Answer from the drawing. Dimensions are ordinates in mm from the lowest x, y and z of the part. A direction names the side the tool comes from. Coordinates: 2 decimals unless noted, no trailing zeros. Loops run counter-clockwise (first coordinate to the right, second up) from the corner with the lowest first, then second, coordinate; pieces in that order, holes last. Notation, with made-up numbers: M 10,39.25 L 69,39.25 A16 ccw 69,63.25 Z; hole C 19,41 d5. An arc over 180 degrees is marked long. Put each result on its own line as item: value.
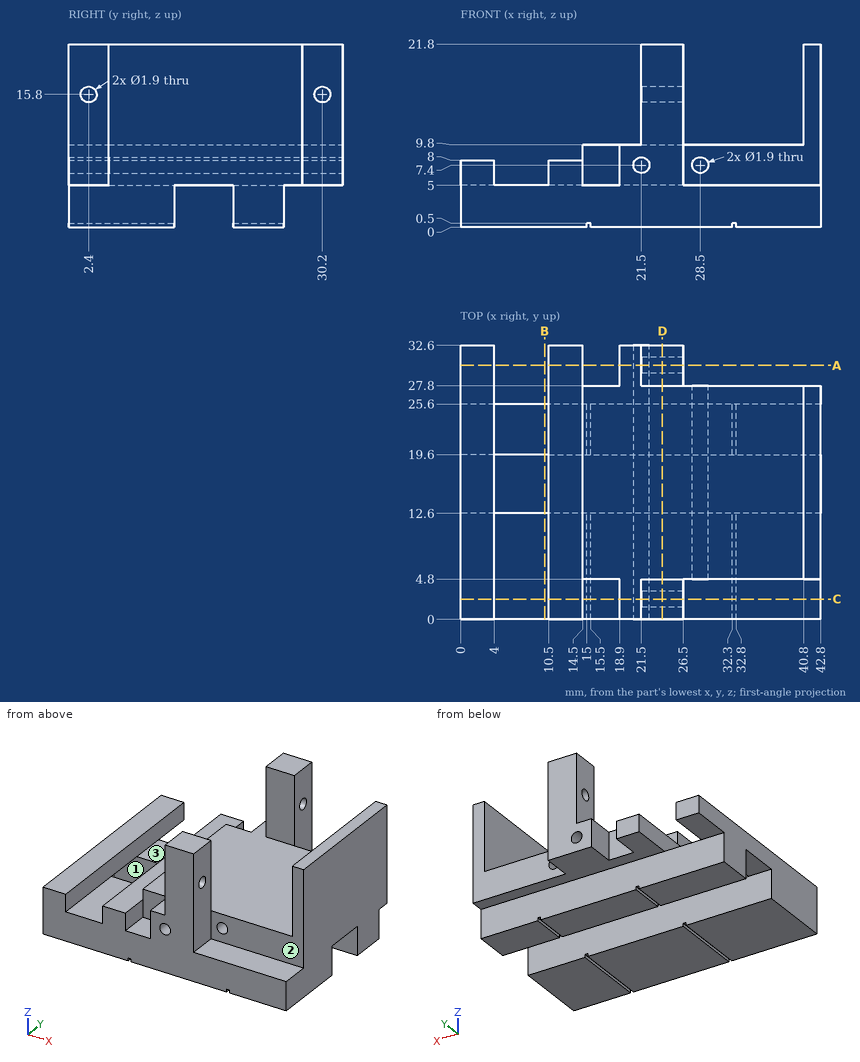
1) Find section C-C, the plane y = 2.4. Count the separate pieces of the cut face and the enclosed holes in it, plus the area to 3 significant figures.
Answer list:
separate pieces: 2
enclosed holes: 1
area: 322 mm^2
2) Find section D-D, the plane x = 24. Write down the section's boundary in (y, z), plus the area to 3 significant figures.
Answer list:
outline: M 0,0 L 12.6,0 L 12.6,5 L 19.6,5 L 19.6,0 L 25.6,0 L 25.6,5 L 32.6,5 L 32.6,21.8 L 27.8,21.8 L 27.8,9.8 L 4.8,9.8 L 4.8,21.8 L 0,21.8 Z; hole C 2.4,15.8 d1.9; hole C 30.2,15.8 d1.9
area: 359 mm^2
3) Find section A-A, the plane y = 30.2. Write down the section's boundary in (x, z).
Answer list:
outline: M 0,5 L 4,5 L 4,8 L 0,8 Z; M 10.5,5 L 14.5,5 L 14.5,8 L 10.5,8 Z; M 18.9,5 L 26.5,5 L 26.5,14.85 L 21.5,14.85 L 21.5,9.8 L 18.9,9.8 Z; M 21.5,16.75 L 26.5,16.75 L 26.5,21.8 L 21.5,21.8 Z; hole C 21.5,7.4 d1.9
4) Given pin 1 Ø6.5 at (x, y) = (6.5, 22.5) entering from +Z; pin 2 Ø4 at (y, z) = (30, 18.5) entering from -X; pin 3 Ø1.5 at (x, z) = (21.5, 7.4) entering from +Y; pin 4 Ø1.5 at (x, y) = (15.5, 21.5) entering from +Z, each flat-ended and moving along its own axis, determine where each tip first touches the part or whether it passes through.
Answer list:
pin 1: stops at z = 8
pin 2: stops at x = 21.5
pin 3: passes through
pin 4: stops at z = 9.8
5) Which of the six approach directions +Z, -Z, +X, -X, +Y, -Y give full straight-line access (tool end or side, diameter ignored) to the marked faces 1, 2 and 3?
Answer list:
face 1: -Z, +X, -X
face 2: +Z, +X, -Y
face 3: +Z, +Y, -Y
6) Find section B-B, the plane x = 10. Write down the section's boundary in (y, z).
Answer list:
outline: M 0,0 L 12.6,0 L 12.6,5 L 0,5 Z; M 19.6,0 L 25.6,0 L 25.6,5 L 19.6,5 Z
7) Straight lines are drawn through the part: line 1 (Y direction, x = 25.1, z = 15.8); line 2 (Z direction, x = 21.5, y = 13); line 3 (Y direction, x = 10.5, z = 1.25). For each, find the intervals that lie inside material, in ascending order. Write a range as [from, to].
Answer list:
line 1: y = [0, 1.45], [3.35, 4.8], [27.8, 29.25], [31.15, 32.6]
line 2: z = [5, 6.45], [8.35, 9.8]
line 3: y = [0, 12.6], [19.6, 25.6]
